```python
from build123d import *

# Parameters (mm, degrees)
SKETCH1_W           = 150
SKETCH1_H           = 130
SKETCH1_R           = 1.5
BOSS_EXTRUDE1_DEPTH = 2
SKETCH3_R           = 2.5
BOSS_EXTRUDE2_DEPTH = 1


with BuildPart() as part:
    # Sketch1 → Boss-Extrude1 (new body)
    with BuildSketch(Plane.XY):
        with Locations((-1.886747415, -24.010339734)):
            Rectangle(SKETCH1_W, SKETCH1_H)
        with Locations((-61.886747415, 35.989660266)):
            Circle(SKETCH1_R, mode=Mode.SUBTRACT)
        with Locations((58.113252585, 35.989660266)):
            Circle(SKETCH1_R, mode=Mode.SUBTRACT)
        with Locations((-61.886747415, -24.010339734)):
            Circle(SKETCH1_R, mode=Mode.SUBTRACT)
        with Locations((58.113252585, -24.010339734)):
            Circle(SKETCH1_R, mode=Mode.SUBTRACT)
    extrude(amount=BOSS_EXTRUDE1_DEPTH)

    # Sketch3 → Boss-Extrude2 (add)
    with BuildSketch(Plane.XY.offset(2)):
        with Locations((-4.64809573, -79.010339734)):
            Circle(SKETCH3_R)
        with BuildLine():
            ThreePointArc((6.923235342, -72.232974628), (-5.323558957, -66.063152089), (-17.570353256, -72.232974628))
            ThreePointArc((-17.570353256, -72.232974628), (-17.211884144, -74.638125217), (-14.806733555, -74.279656105))
            ThreePointArc((-14.806733555, -74.279656105), (-5.323558957, -69.502119801), (4.159615641, -74.279656105))
            ThreePointArc((4.159615641, -74.279656105), (6.56476623, -74.638125217), (6.923235342, -72.232974628))
        make_face()
        with BuildLine():
            ThreePointArc((18.078397342, -62.968741701), (-4.900318567, -52.033991798), (-27.879034477, -62.968741701))
            ThreePointArc((-27.879034477, -62.968741701), (-27.581012613, -65.854503882), (-24.695250433, -65.556482018))
            ThreePointArc((-24.695250433, -65.556482018), (-4.900318567, -56.136781189), (14.894613298, -65.556482018))
            ThreePointArc((14.894613298, -65.556482018), (17.780375479, -65.854503882), (18.078397342, -62.968741701))
        make_face()
        with BuildLine():
            ThreePointArc((13.443037293, -67.850100594), (-5.007901344, -58.749928764), (-23.458839981, -67.850100594))
            ThreePointArc((-23.458839981, -67.850100594), (-23.164962626, -70.080553699), (-20.934509521, -69.786676345))
            ThreePointArc((-20.934509521, -69.786676345), (-5.007901344, -61.931527405), (10.918706833, -69.786676345))
            ThreePointArc((10.918706833, -69.786676345), (13.149159939, -70.080553699), (13.443037293, -67.850100594))
        make_face()
    extrude(amount=BOSS_EXTRUDE2_DEPTH)


solid = part.part
```
For this review, take the finished solid that the model builds, in its own axes (mm). A direction names the side the tool comes from. Coordinates: 2 decimals unless noted, no trailing zeros. Loops run counter-clockwise (first coordinate to the right, second up) from the corner with the lowest first, then second, coordinate; pieces in that order, holes last.
1. Insertion check: P1, Ø8, axis at x = 33.5, y = 0.5, coming from the +Z side; P2, Ø2.5, axis at x = 58.11, y = 35.99, coming from the +Z side. Each pin has a flat end and moves straight along its axis. Give the tip position at first contact, or say it passes through.
2. Add section B-B, the plane x = -9.5. Give the boundary of the cut face in (y, z), then the cut area to 3 significant figures.
3. Add section A-A, the plane y = -13. Give the boundary of the cut face in (x, z), then the cut area to 3 significant figures.
4. For line 1 (Y direction, x = -63, z = 1.1); line 2 (Z direction, x = -55.5, y = 24.5); line 3 (Y direction, x = -2, z = 2.5), list the stretches that pass through material, from the lowest coordinate up.
5. Add section C-C, the plane x = 55. Give the boundary of the cut face in (y, z).
6. For faces 1 (the cylindrical face through (-5.22, -56.14, 2.49)), 2 (the flat face through (-5.01, -55.97, 3)), 3 (the cylindrical face through (-4.532, -52.036, 2.493)), list the 3-axis set-ups (+Z, -Z, +X, -X, +Y, -Y) from which the entire face can be reached by the end or side of a thin tool; tool diameter is ignored.
7. Mouldability with a two-part tool opening along Y and no side actions: class faces 4 (the cylindrical face through (-5.124, -66.064, 2.493)), 5 (the cylindrical face through (-5.478, -69.503, 2.493)), 6 (the flat face through (-3, -23, 0)), 7 (the cylindrical face through (-27.616, -65.826, 2.493)) as +Y half, -Y half, draft (parallel to the pull), parting line (faces both ways), or undercut.
Result:
1. P1: stops at z = 2
1. P2: passes through
2. outline: (-89.01, 0) - (40.99, 0) - (40.99, 2) - (-52.39, 2) - (-52.39, 3) - (-56.55, 3) - (-56.55, 2) - (-59.19, 2) - (-59.19, 3) - (-62.44, 3) - (-62.44, 2) - (-66.65, 2) - (-66.65, 3) - (-70.27, 3) - (-70.27, 2) - (-89.01, 2) - close
2. area: 271 mm2
3. outline: (-76.89, 0) - (73.11, 0) - (73.11, 2) - (-76.89, 2) - close
3. area: 300 mm2
4. line 1: y = -89.01 to -25.02, -23.01 to 34.98, 36.99 to 40.99
4. line 2: z = 0 to 2
4. line 3: y = -69.98 to -66.43, -62.16 to -58.95, -56.3 to -52.18
5. outline: (-89.01, 0) - (40.99, 0) - (40.99, 2) - (-89.01, 2) - close
6. face 1: +Z
6. face 2: +Z, +X, -X, +Y, -Y
6. face 3: +Z, +Y
7. face 4: undercut
7. face 5: undercut
7. face 6: draft
7. face 7: parting line
